Here's the drawing with two shaded views (mm, measured from the low corner). I have some questions. A direction names the side the tool comes from. Give positions to 0.01 mm unless a question says otherwise; leave off trailing zeros. Write each loop counter-clockwise with the first axis right and the second up, starting at its lowest first coordinate (ties: lowest second). Pieces come first, ordered by that corner, then holes.
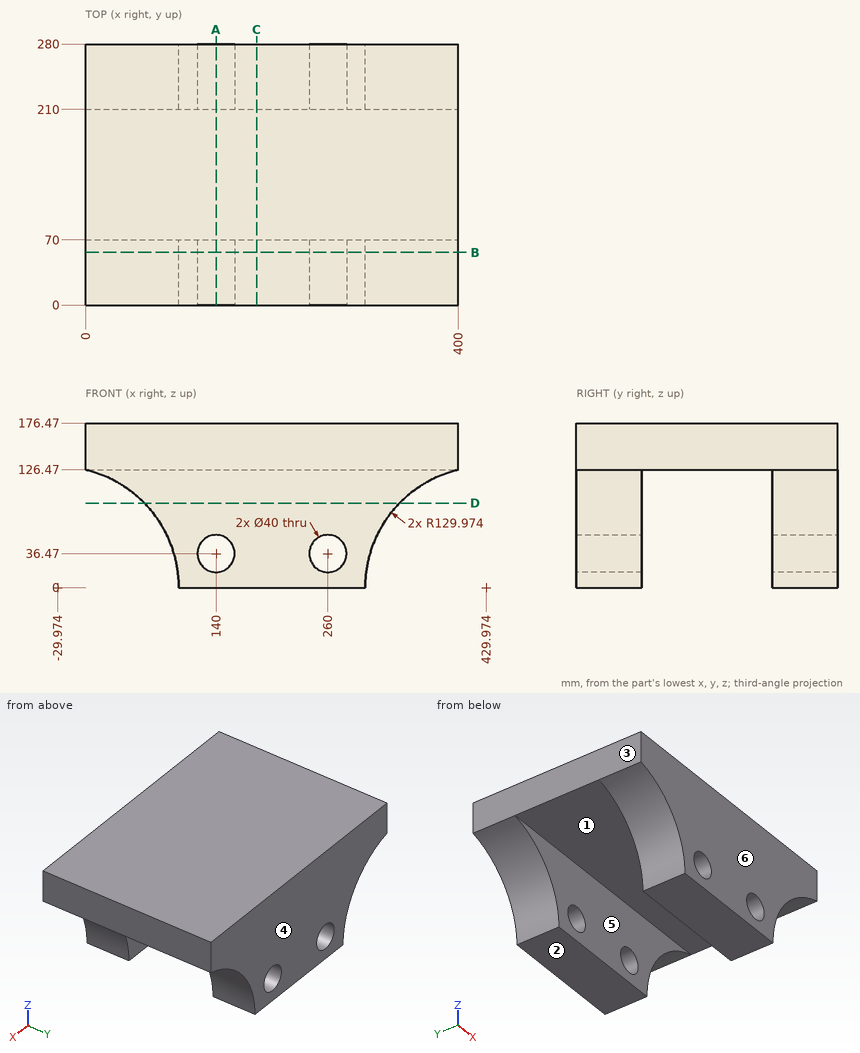
1) Please list where these lines run through material, in increasing order: L1, parallel to Z at x = 140, y = 42; L2, parallel to X at y = 23, z = 53 (1 decimal); L3, parallel to Y at x = 303.5, z = 66.
Values follow:
L1: z = 0 to 16.47, 56.47 to 176.47
L2: x = 88.7 to 128.7, 151.3 to 248.7, 271.3 to 311.3
L3: y = 0 to 70, 210 to 280
2) For pin 1 Ø2 at (x, y) = (42.5, 151.5) entering from -Z; pin 2 Ø24 at (x, z) = (140, 36.47) entering from +Y, each with a flat end and sliding along its axis, tell me the tip position at first contact or that it passes through.
Values follow:
pin 1: stops at z = 126.47
pin 2: passes through
3) For the marked faces 1 and 2, which set-ups out of +Z, -Z, +X, -X, +Y, -Y let a thin tool reach every point of the face, with its end or its side?
Values follow:
face 1: -Z, +X, -X
face 2: -Z, +X, -X, +Y, -Y
4) If we mould it in two halves opening along Y, with no side actions, what happens to the marked faces 3, 4, 5 and 6? For each: +Y half, -Y half, draft (parallel to the pull), parting line (faces both ways), or undercut.
Values follow:
face 3: draft
face 4: +Y half
face 5: undercut
face 6: -Y half
5) Suppose I cut it at A-A on x = 140. Write out the boundary of the cut face in (y, z), plus the area to 3 significant figures.
Values follow:
outline: (0, 0) - (70, 0) - (70, 16.47) - (0, 16.47) - close; (0, 56.47) - (70, 56.47) - (70, 126.47) - (210, 126.47) - (210, 56.47) - (280, 56.47) - (280, 176.47) - (0, 176.47) - close; (210, 0) - (280, 0) - (280, 16.47) - (210, 16.47) - close
area: 26,100 mm2
6) Suppose I cut it at D-D on z = 90.5. Write out the boundary of the cut face in (x, y) (1 decimal).
Values follow:
outline: (63.3, 0) - (336.7, 0) - (336.7, 70) - (63.3, 70) - close; (63.3, 210) - (336.7, 210) - (336.7, 280) - (63.3, 280) - close
7) Suppose I cut it at B-B on y = 56.5. Write out the boundary of the cut face in (x, z).
Values follow:
outline: (0, 126.47) arc R129.97 cw to (100, 0) - (300, 0) arc R129.97 cw to (400, 126.47) - (400, 176.47) - (0, 176.47) - close; hole circle Ø40 at (140, 36.47); hole circle Ø40 at (260, 36.47)
8) Suppose I cut it at C-C on x = 183.5. Write out the boundary of the cut face in (y, z).
Values follow:
outline: (0, 0) - (70, 0) - (70, 126.47) - (210, 126.47) - (210, 0) - (280, 0) - (280, 176.47) - (0, 176.47) - close
